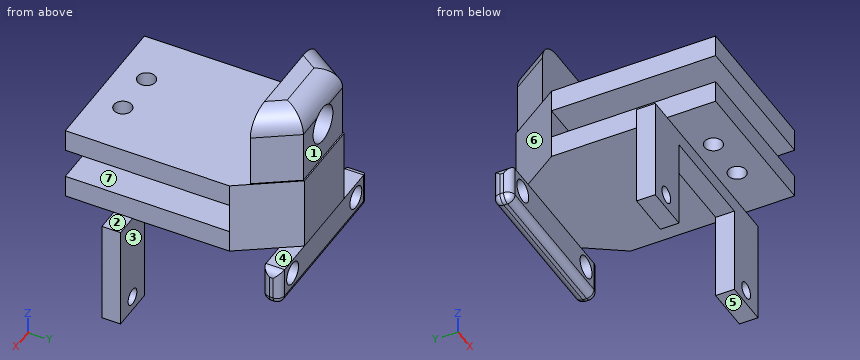
from build123d import *

# Parameters (mm, degrees)
SKETCH_R        = 1.2
PAD_DEPTH       = 3
PAD001_DEPTH    = 10
FILLET_R        = 3
SKETCH002_R     = 2.5
POCKET_DEPTH    = 6
SKETCH003_R     = 1.2
PAD002_DEPTH    = 7
SKETCH004_W     = 20
SKETCH004_H     = 4
POCKET001_DEPTH = 22
PAD003_DEPTH    = 14
SKETCH006_R     = 1.1
POCKET002_DEPTH = 3
PAD004_DEPTH    = 5
SKETCH008_R     = 1.5
POCKET003_DEPTH = 5
FILLET001_R     = 1
POCKET004_DEPTH = 5


with BuildPart() as part:
    # Sketch → Pad (new body)
    with BuildSketch(Plane.XY):
        Polygon((-20, 22), (-20, 0), (0, 0), (0, 22), (-5, 29.412805), (-15, 29.412805), align=None)
        with Locations((-7, 4)):
            Circle(SKETCH_R, mode=Mode.SUBTRACT)
        with Locations((-13, 4)):
            Circle(SKETCH_R, mode=Mode.SUBTRACT)
    extrude(amount=PAD_DEPTH)

    # Sketch001 (on Face10 of Pad) → Pad001 (join)
    with BuildSketch(Plane.XY.offset(3)):
        Polygon((-10, 24), (-1.5, 24), (-5.038419, 29.245922), (-14.961581, 29.245922), (-18.5, 24), align=None)
    extrude(amount=PAD001_DEPTH)

    # Fillet
    fillet_edges = [part.edges().sort_by_distance(p)[0] for p in [
        (-3.26921, 26.622961, 13),
        (-10, 29.245922, 13),
        (-16.73079, 26.622961, 13),
    ]]
    fillet(fillet_edges, radius=FILLET_R)

    # Sketch002 (on Face1 of Fillet) → Pocket (cut)
    with BuildSketch(Plane.XZ.offset(-24)):
        with Locations((-10, 8)):
            Circle(SKETCH002_R)
    extrude(amount=-POCKET_DEPTH, mode=Mode.SUBTRACT)

    # Sketch003 (on Face20 of Pocket) → Pad002 (join)
    with BuildSketch(Plane(origin=(0, 0, 0), x_dir=(1, 0, 0), z_dir=(0, 0, -1))):
        Polygon((0, 0), (-20, 0), (-20, -22), (-15, -29.412805), (-5, -29.412805), (0, -22), align=None)
        with Locations((-13, -4)):
            Circle(SKETCH003_R, mode=Mode.SUBTRACT)
        with Locations((-7, -4)):
            Circle(SKETCH003_R, mode=Mode.SUBTRACT)
    extrude(amount=PAD002_DEPTH)

    # Sketch004 (on Face22 of Pad002) → Pocket001 (cut)
    with BuildSketch(Plane.XZ):
        with Locations((-10, -2)):
            Rectangle(SKETCH004_W, SKETCH004_H)
    extrude(amount=-POCKET001_DEPTH, mode=Mode.SUBTRACT)

    # Sketch005 (on Face26 of Pocket001) → Pad003 (join)
    with BuildSketch(Plane(origin=(0, 0, -7), x_dir=(1, 0, 0), z_dir=(0, 0, -1))):
        Polygon((-10, -6.5), (-23, -6.5), (-23, -9), (-10, -9), (3, -9), (3, -6.5), align=None)
    extrude(amount=PAD003_DEPTH)

    # Sketch006 (on Face33 of Pad003) → Pocket002 (cut)
    with BuildSketch(Plane(origin=(0, 9, 0), x_dir=(-1, 0, 0), z_dir=(0, 1, 0))):
        with Locations((0, -19)):
            Circle(SKETCH006_R)
        with Locations((20.2, -19)):
            Circle(SKETCH006_R)
    extrude(amount=-POCKET002_DEPTH, mode=Mode.SUBTRACT)

    # Sketch007 (on Face26 of Pocket002) → Pad004 (join)
    with BuildSketch(Plane(origin=(0, 0, -7), x_dir=(1, 0, 0), z_dir=(0, 0, -1))):
        Polygon((-10, -26.9), (-21, -26.9), (-21, -29.4), (-10, -29.4), (1, -29.4), (1, -26.9), align=None)
    extrude(amount=PAD004_DEPTH)

    # Sketch008 → Pocket003 (cut)
    with BuildSketch(Plane(origin=(0, 29.4, 0), x_dir=(-1, 0, 0), z_dir=(0, 1, 0))):
        with Locations((2.021394, -9)):
            Circle(SKETCH008_R)
        with Locations((18.020098, -9)):
            Circle(SKETCH008_R)
    extrude(amount=-POCKET003_DEPTH, mode=Mode.SUBTRACT)

    # Fillet001
    fillet001_edges = [part.edges().sort_by_distance(p)[0] for p in [
        (-21, 26.9, -9.5),
        (-21, 29.4, -9.5),
        (-21, 28.15, -7),
        (-21, 28.15, -12),
        (-4.5, 29.4, -12),
        (-15.5, 29.4, -12),
        (-15.5, 26.9, -12),
        (-4.5, 26.9, -12),
        (1, 29.4, -9.5),
        (1, 26.9, -9.5),
        (1, 28.15, -12),
        (1, 28.15, -7),
    ]]
    fillet(fillet001_edges, radius=FILLET001_R)

    # Sketch009 (on Face29 of Fillet001) → Pocket004 (cut)
    with BuildSketch(Plane(origin=(0, 9, 0), x_dir=(-1, 0, 0), z_dir=(0, 1, 0))):
        Polygon((3, -15), (3, -21), (17, -21), (17, -9), (3, -9), align=None)
    extrude(amount=-POCKET004_DEPTH, mode=Mode.SUBTRACT)


solid = part.part
Geometry check sheet. Reference: the model listing, model coordinates, mm. Face numbers are marked on the shaded views. A direction names the side the tool comes from. Give positions to 0.01 mm unless a question says otherwise; leave off trailing zeros. Write each loop counter-clockwise with the first axis right and the second up, starting at its lowest first coordinate (ties: lowest second). Pieces come first, ordered by that corner, then holes.
1) Cross-section at B-B (z = -14). Record the boundary of the cut face in (x, y).
Values follow:
outline: (-23, 6.5) - (-17, 6.5) - (-17, 9) - (-23, 9) - close; (-3, 6.5) - (3, 6.5) - (3, 9) - (-3, 9) - close
2) Cross-section at C-C (y = 8). Record the boundary of the cut face in (x, z), plus the area to 3 significant figures.
Values follow:
outline: (-23, -21) - (-17, -21) - (-17, -9) - (-3, -9) - (-3, -21) - (3, -21) - (3, -7) - (0, -7) - (0, -4) - (-20, -4) - (-20, -7) - (-23, -7) - close; (-20, 0) - (0, 0) - (0, 3) - (-20, 3) - close; hole circle Ø2.2 at (-20.2, -19); hole circle Ø2.2 at (0, -19)
area: 308 mm2
3) Go/stop test with flat-tipped pins: pin 1 Ø3 at (x, z) = (-12.5, -9) entering from -Y; pin 2 Ø1 at (x, y) = (-12, 24) entering from -Z; pin 3 Ø0.9 at (y, z) = (9, 1) entering from +X. Record where each tip stops, or that it passes through.
Values follow:
pin 1: stops at y = 6.5
pin 2: stops at z = -7
pin 3: stops at x = 0
4) Cross-section at A-A (y = 13). Record the boundary of the cut face in (x, z).
Values follow:
outline: (-20, -7) - (0, -7) - (0, -4) - (-20, -4) - close; (-20, 0) - (0, 0) - (0, 3) - (-20, 3) - close
5) Set-up check for the marked faces 1, 2 and 3: record each of +Z, -Z, +X, -X, +Y, -Y from which the full face is reachable in a straight line by a thin tool's end or side.
Values follow:
face 1: +Z, +X, -X, +Y
face 2: +Z, +X, +Y, -Y
face 3: -Z, +X, -X
6) Thickness scan on line 1 (Z direction, x = -3.5, y = 5.5); line 2 (Y direction, x = -19.25, z = -8); line 3 (Z direction, x = -8.75, y = 8). Record the ranges inside material, lowest first.
Values follow:
line 1: z = -7 to -4, 0 to 3
line 2: y = 6.5 to 9, 26.9 to 29.4
line 3: z = -9 to -4, 0 to 3
7) Release check for a two-part mould opening along Z. For the marked faces 4, 5, 6 and 7 record: released by +Z, released by -Z, zero draft, split by the parting line, or undercut.
Values follow:
face 4: released by +Z
face 5: released by -Z
face 6: zero draft
face 7: undercut
